Part model, mm, in its own coordinate system. A direction names the side the tool comes from. Give positions to 0.01 mm unless a question says otherwise; leave off trailing zeros. Write each loop counter-clockwise with the first axis right and the second up, starting at its lowest first coordinate (ties: lowest second). Pieces come first, ordered by that corner, then holes. Notation, with made-up numbers: M 30,18.25 L 66,18.25 A14 ccw 66,24.25 Z; hole C -31.5,76 d6. An arc over 180 degrees is marked long. Answer as CSV lines item,"result". Start each with the question number.
Item 1: Band-saw the part on A-A, the plane y = 6. List the corners of the cut face in (x, z).
Item 2: Wall check: L1, parallel to Y at x = 5, z = 1.35; L2, parallel to Y at x = -35, z = 8; L3, parallel to X at y = -33.75, z = 4.15. Give the ranges that are in metal, low to high. Write a range as from..to.
Item 3: Band-saw the part on C-C, the plane z = 23.5. List the corners of the cut face in (x, y), then the cut area to 3 significant figures.
Item 4: Two-plate mould, pull along Y, no slides. Class faces 1 (the flat face through (-15, -23, 45)), 2 (the cylindrical face through (-38.966, 34.271, 7.972)), 3 (the flat face through (-1, 40, 5)): +Y half, -Y half, draft (parallel to the pull), parting line (faces both ways), or undercut.
Item 5: 3-axis set-ups, long thin cutter, end or side, ignore diameter. For faces 4 (the cylindrical face through (4.324, 31.604, 2.958)), 5 (the flat face through (-40, 0, 17)), 6 (the flat face through (-15, 27.5, 32)), 7 (the flat face through (-14, 22.5, 32)), 8 (the flat face through (-32.5, -23, 32)): which of +Z, -Z, +X, -X, +Y, -Y reach the whole face in a straight line?
Item 6: Band-saw the part on D-D, the plane x = 5. Count the separate pieces of the cut face and the enclosed holes in it, then the cut area to 3 significant figures.
Item 7: Band-saw the part on B-B, the plane x = -28.5. List the corners of the cut face in (y, z).
Item 8: Pin check, flat tips, straight feed: pin 1 (8 mm diameter, centred on x = -24.5, z = 16, fed in from +Y); pin 2 (10.5 mm diameter, centred on y = 9.5, z = 36, fed in from -X); pin 3 (7 mm diameter, centred on x = 5, y = 33.75, fed in from +Z). Stop position of each tip, or through.
Autodesk Inventor part; units mm, degrees
ref_plane "YZ Plane" through (0, 0, 0) normal (1, 0, 0) x (0, 1, 0)
ref_plane "XZ Plane" through (0, 0, 0) normal (0, 1, 0) x (-1, 0, 0)
ref_plane "XY Plane" through (0, 0, 0) normal (0, 0, 1) x (1, 0, 0)
sketch "Sketch1" plane through (0, 0, 0) normal (0, 0, 1) x (1, 0, 0)
  line L0 (-42.5, 40) -> (42.5, 40)
  line L1 (42.5, 40) -> (42.5, -40)
  line L2 (42.5, -40) -> (-42.5, -40)
  line L3 (-42.5, -40) -> (-42.5, 40)
  point P0 (0, 0)
  dimension "d0" = 85
  dimension "d1" = 42.5
  dimension "d2" = 80
  dimension "d3" = 40
extrude "Extrusion1" add sketch "Sketch1" along normal blind 10
sketch "Sketch2" plane through (0, 0, 10) normal (0, 0, 1) x (1, 0, 0)
  line L0 (-42.5, 40) -> (-42.5, -40)
  point P0 (0, 0)
  point P1 (-35, -33.75)
  point P2 (5, -33.75)
  point P3 (-35, 33.75)
  point P4 (5, 33.75)
  dimension "d6" = 40
  dimension "d7" = 67.5
  dimension "d8" = 33.75
  dimension "d9" = 7.5
hole "Hole1" at (-35, -33.75, 10) at (5, -33.75, 10) at (-35, 33.75, 10) at (5, 33.75, 10) direction (0, 0, -1) diameter 4.5 end through all counterbore diameter 8 counterbore depth 4
sketch "Sketch3" plane through (0, 0, 10) normal (0, 0, 1) x (1, 0, 0)
  line L0 (-42.5, 27.5) -> (13.5, 27.5)
  line L1 (13.5, 27.5) -> (13.5, -27.5)
  line L2 (13.5, -27.5) -> (-42.5, -27.5)
  line L3 (-42.5, -27.5) -> (-42.5, 27.5)
  line L4 (-42.5, 40) -> (-42.5, -40)
  line L5 (-35, 22.5) -> (8.5, 22.5)
  line L6 (8.5, 22.5) -> (8.5, -20)
  line L7 (8.5, -20) -> (-35, -20)
  line L8 (-35, -20) -> (-35, 22.5)
  point P0 (0, 0)
  dimension "d17" = 56
  dimension "d18" = 55
  dimension "d19" = 27.5
  dimension "d20" = 5
  dimension "d21" = 5
  dimension "d22" = 7.5
  dimension "d23" = 7.5
extrude "Extrusion2" add sketch "Sketch3" along normal blind 45
sketch "Sketch4" plane through (-42.5, -27.5, 10) normal (0, -1, 0) x (1, 0, 0)
  line L0 (5, 40) -> (51, 40)
  line L1 (51, 40) -> (51, 5)
  line L2 (51, 5) -> (5, 5)
  line L3 (5, 5) -> (5, 40)
  line L4 (0, 0) -> (0, 45)
  line L5 (56, 0) -> (56, 45)
  line L6 (51, 45) -> (7.5, 45)
  line L7 (0, 0) -> (85, 0)
  point P0 (42.5, -10)
  dimension "d27" = 5
  dimension "d28" = 5
  dimension "d29" = 5
  dimension "d30" = 5
extrude "Extrusion3" cut sketch "Sketch4" against normal blind 2.5
sketch "Sketch5" plane through (-42.5, -25, 10) normal (0, -1, 0) x (1, 0, 0)
  line L0 (10, 35) -> (46, 35)
  line L1 (46, 35) -> (46, 10)
  line L2 (46, 10) -> (10, 10)
  line L3 (10, 10) -> (10, 35)
  line L4 (5, 40) -> (51, 40)
  line L5 (5, 5) -> (5, 40)
  line L6 (51, 5) -> (5, 5)
  line L7 (51, 40) -> (51, 5)
  point P0 (42.5, -10)
  dimension "d33" = 5
  dimension "d34" = 5
  dimension "d35" = 5
  dimension "d36" = 5
extrude "Extrusion4" cut sketch "Sketch5" against normal up to surface (5 mm away) contours L0 L1 L2 L3
sketch "Sketch6" plane through (-42.5, -40, 0) normal (-1, 0, 0) x (0, 0, 1)
  line L0 (50, 62.5) -> (15, 62.5)
  line L1 (15, 62.5) -> (15, 17.5)
  line L2 (15, 17.5) -> (50, 17.5)
  line L3 (50, 17.5) -> (50, 62.5)
  line L4 (55, 67.5) -> (55, 12.5)
  line L5 (10, 67.5) -> (55, 67.5)
  line L6 (10, 80) -> (10, 67.5)
  line L7 (10, 12.5) -> (55, 12.5)
  point P0 (0, 40)
  dimension "d39" = 5
  dimension "d40" = 5
  dimension "d41" = 5
  dimension "d42" = 5
extrude "Extrusion5" cut sketch "Sketch6" against normal blind 2.5
sketch "Sketch7" plane through (-40, -40, 0) normal (-1, 0, 0) x (0, 0, 1)
  line L0 (45, 57.5) -> (20, 57.5)
  line L1 (20, 57.5) -> (20, 22.5)
  line L2 (20, 22.5) -> (45, 22.5)
  line L3 (45, 22.5) -> (45, 57.5)
  line L4 (50, 62.5) -> (50, 17.5)
  line L5 (50, 17.5) -> (15, 17.5)
  line L6 (15, 17.5) -> (15, 62.5)
  line L7 (15, 62.5) -> (50, 62.5)
  point P0 (0, 40)
  dimension "d45" = 5
  dimension "d46" = 5
  dimension "d47" = 5
  dimension "d48" = 5
extrude "Extrusion6" cut sketch "Sketch7" against normal up to surface (5 mm away) contours L3 L2 L1 L0
equation "\"d21\" = d20"
properties part number "sampleChamber_singlePiece"
Output:
1,outline,"M -42.5,0 L 42.5,0 L 42.5,10 L 13.5,10 L 13.5,55 L 8.5,55 L 8.5,10 L -35,10 L -35,20 L -40,20 L -40,15 L -42.5,15 Z; M -42.5,50 L -40,50 L -40,45 L -35,45 L -35,55 L -42.5,55 Z"
2,L1,"-40..-36, -31.5..31.5, 36..40"
2,L2,"-40..-37.75, -29.75..29.75, 37.75..40"
2,L3,"-42.5..-37.25, -32.75..2.75, 7.25..42.5"
3,outline,"M -42.5,-27.5 L -37.5,-27.5 L -37.5,-25 L -32.5,-25 L -32.5,-20 L -35,-20 L -35,-17.5 L -40,-17.5 L -40,-22.5 L -42.5,-22.5 Z; M -42.5,22.5 L -40,22.5 L -40,17.5 L -35,17.5 L -35,22.5 L 8.5,22.5 L 8.5,-20 L 3.5,-20 L 3.5,-25 L 8.5,-25 L 8.5,-27.5 L 13.5,-27.5 L 13.5,27.5 L -42.5,27.5 Z"
3,area,"649 mm²"
4,face 1,"draft"
4,face 2,"undercut"
4,face 3,"+Y half"
5,face 4,"+Z, -Z"
5,face 5,"-X"
5,face 6,"+Z, +X, -X, +Y"
5,face 7,"+Z"
5,face 8,"-Y"
6,separate pieces,"3"
6,enclosed holes,"0"
6,area,"1,160 mm²"
7,outline,"M -40,0 L 40,0 L 40,10 L 27.5,10 L 27.5,55 L 22.5,55 L 22.5,10 L -20,10 L -20,20 L -25,20 L -25,15 L -27.5,15 L -27.5,10 L -40,10 Z; M -27.5,50 L -25,50 L -25,45 L -20,45 L -20,55 L -27.5,55 Z"
8,pin 1,"y = 27.5"
8,pin 2,"x = 8.5"
8,pin 3,"z = 6"
